The model under review builds one solid part; all positions refer to its coordinate system, in mm. A direction names the side the tool comes from. Coordinates: 2 decimals unless noted, no trailing zeros. Order: outer loops, then holes, each group sorted by start corner. A loop starts at its lowest first (then second) coordinate and runs counter-clockwise, first axis right, second up. Notation, with made-up numbers: M 64,-38.75 L 93,-38.75 A23 ccw 93,-16.75 Z; hole C -30,51 d4. An arc over 180 degrees is marked long. Answer as CSV lines item,"result". Start each with the question number.
Q1. Consider section D-D on y = -3.5. Write out the cut boundary in (x, z).
Q2. For P1, Ø5, axis at y = -3, z = -22, coming from the -X side; P2, Ø1, axis at x = -3.5, z = -24.5, coming from the -Y side; P3, Ø5, axis at x = -2.5, z = -25, coming from the -Y side, all flat-tipped, find the tip position at first contact; note any pin that passes through.
Q3. Consider section A-A on y = 0. Write out the cut boundary in (x, z).
Q4. Machinability: for faces 4 (the face through (3, -1, -35)), 5 (the face through (-1.42, -3.92, -1)), which of the approach directions +Z, -Z, +X, -X, +Y, -Y give a long, thin tool a straight path to every point of the face, cutting with its end or side? Answer none if there is none.
Q5. The part is to be moulded in two halves that separate along Y. For faces 1 (the face through (-0.596, -2.685, -17.255)), 2 (the face through (-0.867, 3.905, -17.762)), 3 (the face through (3, -1, 0)), say which applies: +Y half, -Y half, draft (parallel to the pull), parting line (faces both ways), or undercut.
Q6. Wall thickness on L1, parallel to Y at x = 0, z = -9; L2, parallel to Z at x = -4.75, y = -0.5; L3, parallel to X at y = -2.25, z = -17.5: over which ranges is each line inside the solid? List them lowest first. Write a range as [from, to].
Q7. Consider section C-C on z = -9. Write out the cut boundary in (x, y), and give its area (3 significant figures).
from build123d import *

# Parameters (mm, degrees)
F0_R     = 6
F1_DEPTH = 1
F2_R     = 4
F3_DEPTH = 34
F4_R     = 2.75
F5_DEPTH = 35


with BuildPart() as f1:
    # F0 (on Top) → F1 (new body)
    with BuildSketch(Plane.XY):
        Circle(F0_R)
    extrude(amount=-F1_DEPTH)

    # F2 (on face) → F3 (join)
    with BuildSketch(Plane(origin=(0, 0, -1), x_dir=(1, 0, 0), z_dir=(0, 0, -1))):
        Circle(F2_R)
    extrude(amount=F3_DEPTH)

    # F4 (on face) → F5 (cut)
    with BuildSketch(Plane.XY):
        Circle(F4_R)
    extrude(amount=-F5_DEPTH, mode=Mode.SUBTRACT)


solid = f1.part
Evaluation:
1,outline,"M -4.87,-1 L -1.94,-1 L -1.94,-35 L 1.94,-35 L 1.94,-1 L 4.87,-1 L 4.87,0 L -4.87,0 Z"
2,P1,"stops at x = -3.97"
2,P2,"stops at y = -2.65"
2,P3,"stops at y = -4"
3,outline,"M -6,-1 L -4,-1 L -4,-35 L -2.75,-35 L -2.75,0 L -6,0 Z; M 2.75,-35 L 4,-35 L 4,-1 L 6,-1 L 6,0 L 2.75,0 Z"
4,face 4,"-Z, +X, -X, +Y, -Y"
4,face 5,"-Z"
5,face 1,"undercut"
5,face 2,"parting line"
5,face 3,"draft"
6,L1,"y = [-4, -2.75], [2.75, 4]"
6,L2,"z = [-1, 0]"
6,L3,"x = [-3.31, -1.58], [1.58, 3.31]"
7,outline,"C 0,0 d8; hole C 0,0 d5.5"
7,area,"26.5 mm²"
